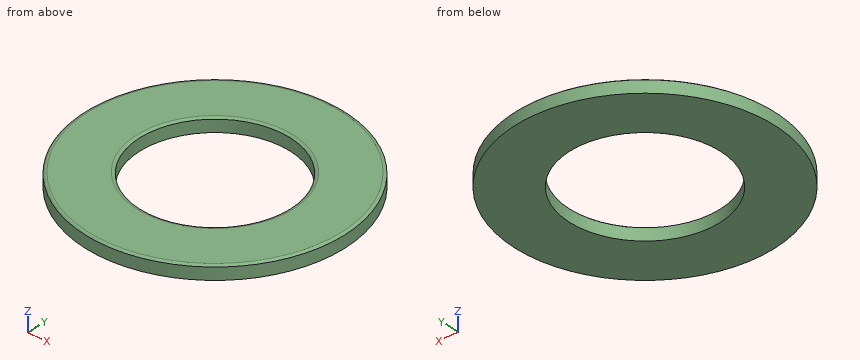
```python
from build123d import *
from OCP.BRepFilletAPI import BRepFilletAPI_MakeChamfer

# Parameters (mm, degrees)
BOSS_EXTRUDE1_START = -1.143
SKETCH3_R           = 22.225
SKETCH3_R_2         = 12.8905
BOSS_EXTRUDE1_DEPTH = 2.286
CHAMFER1_SIZE       = 0.2286
CHAMFER1_SIZE2      = 0.131982272
FILLET1_R           = 0.6858


with BuildPart() as part:
    # Sketch3 → Boss-Extrude1 (new body)
    with BuildSketch(Plane.XY.offset(BOSS_EXTRUDE1_START)):
        Circle(SKETCH3_R)
        Circle(SKETCH3_R_2, mode=Mode.SUBTRACT)
    extrude(amount=BOSS_EXTRUDE1_DEPTH)

    # Chamfer1: one chamfer whose edges measure the first distance from different faces: ONE call of the kernel's chamfer builder (chamfer() names one face for all edges)
    chamfer1_edges_1 = [part.edges().sort_by_distance(p)[0] for p in [
        (-22.225, 0, 1.143),
    ]]
    chamfer1_side_1 = [part.faces().sort_by_distance(p)[0] for p in [
        (-22.225, 0, 0),
    ]]
    chamfer1_edges_2 = [part.edges().sort_by_distance(p)[0] for p in [
        (-12.8905, 0, 1.143),
    ]]
    chamfer1_side_2 = [part.faces().sort_by_distance(p)[0] for p in [
        (-12.8905, 0, 0),
    ]]
    chamfer1 = BRepFilletAPI_MakeChamfer(part.part.solid().wrapped)
    for e in chamfer1_edges_1:
        chamfer1.Add(CHAMFER1_SIZE, CHAMFER1_SIZE2, e.wrapped, chamfer1_side_1[0].wrapped)  # the first distance lies on this face
    for e in chamfer1_edges_2:
        chamfer1.Add(CHAMFER1_SIZE, CHAMFER1_SIZE2, e.wrapped, chamfer1_side_2[0].wrapped)  # the first distance lies on this face
    add(Compound.cast(chamfer1.Shape()), mode=Mode.REPLACE)

    # Fillet1
    # the kernel refuses this fillet: 0.6858 mm, written as the material it takes off along each edge
    with BuildSketch(Plane(origin=(0, 0, 1.143), x_dir=(1, 0, 0), z_dir=(0, -1, 0))) as fillet1_piece_1:
        with BuildLine():
            CenterArc((21.71383486, -0.6858), FILLET1_R, 41.810314896, 48.189685104)
            Line((21.71383486, 0), (21.71383486, 0.013716))
            Line((21.71383486, 0.013716), (22.093017728, 0.013716))
            Line((22.093017728, 0.013716), (22.104896133, 0.006858))
            ThreePointArc((22.104896133, 0.006858), (22.170887269, -0.107442), (22.235223303, -0.219456))
            Line((22.235223303, -0.219456), (22.225, -0.2286))
        make_face()
    revolve(axis=Axis((0, 0, 1.143), (0, 0, 1)), mode=Mode.SUBTRACT)
    with BuildSketch(Plane(origin=(0, 0, 1.143), x_dir=(1, 0, 0), z_dir=(0, -1, 0))) as fillet1_piece_2:
        with BuildLine():
            CenterArc((13.40166514, -0.6858), FILLET1_R, 90, 48.189685104)
            Line((12.8905, -0.2286), (12.880276697, -0.219456))
            ThreePointArc((12.880276697, -0.219456), (12.944612731, -0.107442), (13.010603867, 0.006858))
            Line((13.010603867, 0.006858), (13.022482272, 0.013716))
            Line((13.022482272, 0.013716), (13.40166514, 0.013716))
            Line((13.40166514, 0.013716), (13.40166514, 0))
        make_face()
    revolve(axis=Axis((0, 0, 1.143), (0, 0, 1)), mode=Mode.SUBTRACT)


solid = part.part
```
Read the model definition and answer for the solid it produces. Units are mm, in the model's axes. Give positions to 0.01 mm unless a question says otherwise; leave off trailing zeros. Write each loop counter-clockwise with the first axis right and the second up, starting at its lowest first coordinate (ties: lowest second). Pieces come first, ordered by that corner, then holes. Notation, with made-up numbers: (2, 89) -> (24, 89) arc R18 cw to (24, 115) -> close; hole circle Ø11 at (87.25, 32). An arc over 180 degrees is marked (long way). Answer in a Markdown table with one row per item.
1) Straight lines are drawn through the part: line 1 (Y direction, x = 0, z = -0.6) (1 decimal); line 2 (Y direction, x = 11, z = -0.6); line 3 (X direction, y = -8, z = 0.65). For each, find the intervals that lie inside material, in ascending order. Write a range as [from, to].
Results list:
| item | result |
|---|---|
| line 1 | [-22.2, -12.9], [12.9, 22.2] |
| line 2 | [-19.31, -6.72], [6.72, 19.31] |
| line 3 | [-20.74, -10.11], [10.11, 20.74] |
2) Section A-A on x = 0 is taken. Give the vertices of the cut face in (y, z) (1 decimal), plus the area to 3 significant figures.
Results list:
| item | result |
|---|---|
| outline | (-22.2, -1.1) -> (-12.9, -1.1) -> (-12.9, 0.9) arc R0.7 ccw to (-13.4, 1.1) -> (-21.7, 1.1) arc R0.7 ccw to (-22.2, 0.9) -> close; (12.9, -1.1) -> (22.2, -1.1) -> (22.2, 0.9) arc R0.7 ccw to (21.7, 1.1) -> (13.4, 1.1) arc R0.7 ccw to (12.9, 0.9) -> close |
| area | 42.5 mm^2 |
